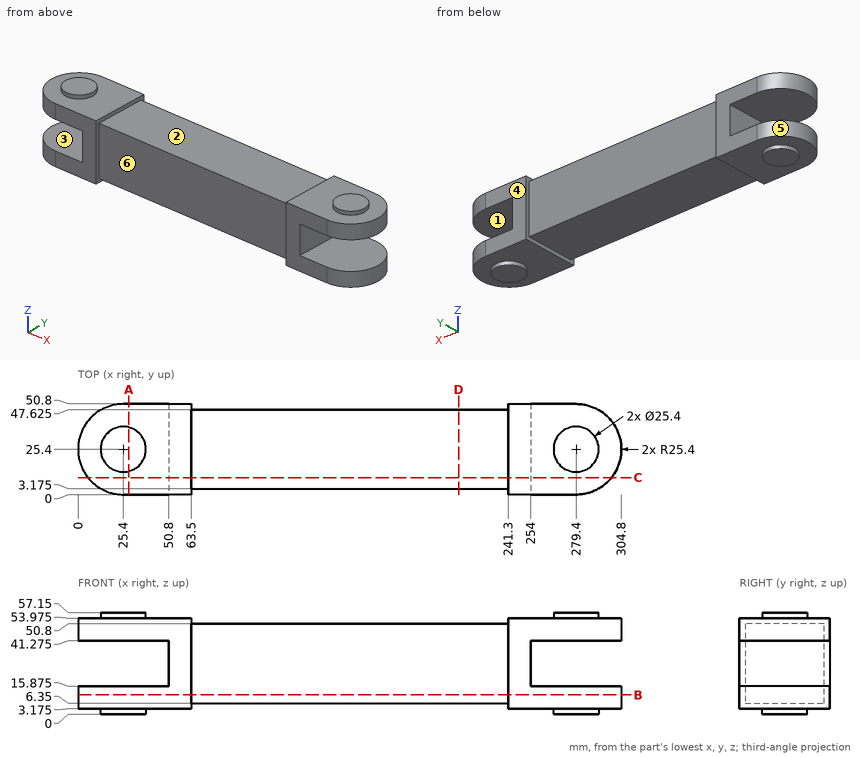
Verification items for this drawing (mm, ordinates from the low corner). A direction names the side the tool comes from. Coordinates: 2 decimals unless noted, no trailing zeros. Order: outer loops, then holes, each group sorted by start corner. A loop starts at its lowest first (then second) coordinate and runs counter-clockwise, first axis right, second up. Notation, with made-up numbers: (-2.5, -19.5) -> (37.5, -19.5) arc R22 cw to (37.5, -4.5) -> close; hole circle Ø10 at (-28, 6). An arc over 180 degrees is marked (long way). Put each result on its own line as item: value. Start each with the question number.
1. Mould release check, pull along X, two halves, no side actions. Record for the marked faces 4, 5 and 6: released by +X, released by -X, zero draft, split by the parting line, or undercut.
2. Cross-section at A-A, the plane x = 28.5. Record the boundary of the cut face in (y, z) (3 decimals), then the cut area to 3 significant figures.
3. Go/stop test with flat-tipped pins: pin 1 Ø12 at (x, y) = (88, 15) entering from -Z; pin 2 Ø13.5 at (x, z) = (195.5, 18) entering from -Y (3 decimals); pin 3 Ø3 at (y, z) = (31.5, 16.5) entering from +X. Record where each tip stops, or that it passes through.
4. Cross-section at B-B, the plane z = 11. Record the boundary of the cut face in (x, y) (3 decimals), then the cut area to 3 significant figures.
5. Access from +Z, -Z, +X, -X, +Y, -Y to the whole of each face (thin tool, end or side, straight path). Record for the marked faces 1, 2 and 3.
6. Cross-section at C-C, the plane y = 9.5. Record the boundary of the cut face in (x, z) (3 decimals), then the cut area to 3 significant figures.
7. Cross-section at D-D, the plane x = 213.5. Record the boundary of the cut face in (y, z) (3 decimals), then the cut area to 3 significant figures.
8. Material ranges on L1, parallel to Z at x = 255.5, y = 42 (3 decimals); L2, parallel to X at y = 41, z = 16; L3, parallel to Z at x = 123, y = 14, recorded low to high. Write a range as [from, to].
Computed:
1. face 4: zero draft
1. face 5: released by -X
1. face 6: undercut
2. outline: (0, 3.175) -> (13.084, 3.175) -> (13.084, 0) -> (37.716, 0) -> (37.716, 3.175) -> (50.8, 3.175) -> (50.8, 15.875) -> (0, 15.875) -> close; (0, 41.275) -> (50.8, 41.275) -> (50.8, 53.975) -> (37.716, 53.975) -> (37.716, 57.15) -> (13.084, 57.15) -> (13.084, 53.975) -> (0, 53.975) -> close
2. area: 1,450 mm2
3. pin 1: z = 6.35
3. pin 2: y = 3.175
3. pin 3: x = 304.35
4. outline: (25.4, 0) -> (63.5, 0) -> (63.5, 3.175) -> (241.3, 3.175) -> (241.3, 0) -> (279.4, 0) arc R25.4 ccw to (279.4, 50.8) -> (241.3, 50.8) -> (241.3, 47.625) -> (63.5, 47.625) -> (63.5, 50.8) -> (25.4, 50.8) arc R25.4 ccw to start
4. area: 13,800 mm2
5. face 1: +X, +Y, -Y
5. face 2: +Z, +Y, -Y
5. face 3: -X, +Y, -Y
6. outline: (5.592, 3.175) -> (63.5, 3.175) -> (63.5, 6.35) -> (241.3, 6.35) -> (241.3, 3.175) -> (299.208, 3.175) -> (299.208, 15.875) -> (254, 15.875) -> (254, 41.275) -> (299.208, 41.275) -> (299.208, 53.975) -> (241.3, 53.975) -> (241.3, 50.8) -> (63.5, 50.8) -> (63.5, 53.975) -> (5.592, 53.975) -> (5.592, 41.275) -> (50.8, 41.275) -> (50.8, 15.875) -> (5.592, 15.875) -> close
6. area: 11,500 mm2
7. outline: (3.175, 6.35) -> (47.625, 6.35) -> (47.625, 50.8) -> (3.175, 50.8) -> close
7. area: 1,980 mm2
8. L1: [3.175, 15.875], [41.275, 53.975]
8. L2: [50.8, 254]
8. L3: [6.35, 50.8]
